Drawing for the job (mm, zero at the part's lowest x, y, z). A direction names the side the tool comes from. Round coordinates to 2 decimals unless told otherwise and drop trailing zeros. Write each loop counter-clockwise with the first axis right and the second up, starting at its lowest first coordinate (ties: lowest second). Pieces come first, ordered by that corner, then holes. Notation, with made-up numbers: M 18.25,72.25 L 48.25,72.25 A9 cw 48.25,87.25 Z; hole C 56,56.5 d5. An arc over 180 degrees is marked long. Use a Markdown table: item, result.
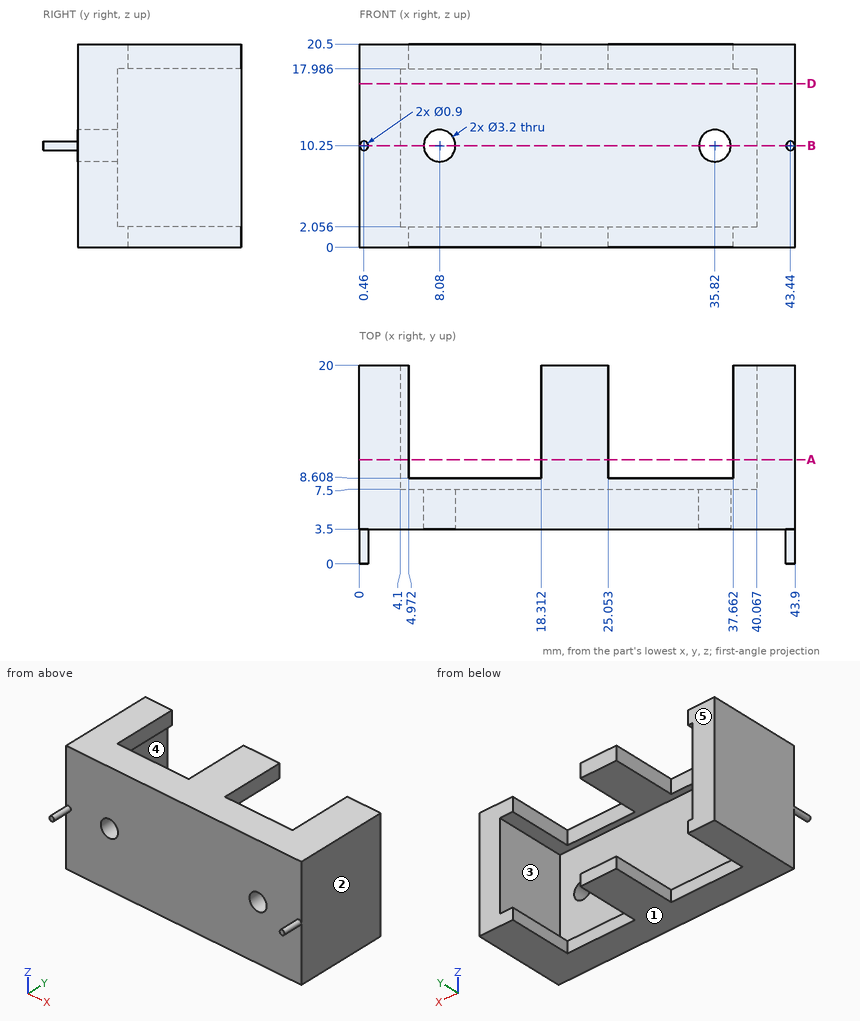
Q1. Cut at A-A on y = 10.5. Give the cut face in (x, z) (1 decimal).
Response values:
| item | result |
|---|---|
| outline | M 0,0 L 5,0 L 5,2.1 L 4.1,2.1 L 4.1,18 L 5,18 L 5,20.5 L 0,20.5 Z; M 18.3,0 L 25.1,0 L 25.1,2.1 L 18.3,2.1 Z; M 18.3,18 L 25.1,18 L 25.1,20.5 L 18.3,20.5 Z; M 37.7,0 L 43.9,0 L 43.9,20.5 L 37.7,20.5 L 37.7,18 L 40.1,18 L 40.1,2.1 L 37.7,2.1 Z |
Q2. Cut at B-B on z = 10.25. Count the separate pieces of the cut face and the enclosed holes in it.
Response values:
| item | result |
|---|---|
| separate pieces | 3 |
| enclosed holes | 0 |
Q3. Cut at D-D on z = 16.5. Give the cut face in (x, y).
Response values:
| item | result |
|---|---|
| outline | M 0,3.5 L 43.9,3.5 L 43.9,20 L 40.07,20 L 40.07,7.5 L 4.1,7.5 L 4.1,20 L 0,20 Z |
Q4. Two-plate mould, pull along Z, no slides. Class the marked faces 1, 2 and 3: +Z half, -Z half, draft (parallel to the pull), parting line (faces both ways), or undercut.
Response values:
| item | result |
|---|---|
| face 1 | -Z half |
| face 2 | draft |
| face 3 | undercut |
Q5. Drill centre lines: L1, parallel to X at y = 6.1, z = 10.25; L2, parallel to X at y = 12, z = 15.25; L3, parallel to Z at x = 39.5, y = 18.75 (1 decimal). Where is each one in solid material? Low to high.
Response values:
| item | result |
|---|---|
| L1 | x = 0 to 6.48, 9.68 to 34.22, 37.42 to 43.9 |
| L2 | x = 0 to 4.1, 40.07 to 43.9 |
| L3 | z = 0 to 2.1, 18 to 20.5 |
Q6. Drop flat-ended pins along their axis: P1, Ø12, axis at x = 24.5, z = 7.5, coming from the -Y side; P2, Ø1.9, axis at x = 8.08, z = 10.25, coming from the -Y side; P3, Ø0.6, axis at x = 9.5, z = 1, coming from the +Y side; P4, Ø5, axis at x = 23.5, z = 13.5, coming from the +Y side. Give the stop position or say it passes through.
Response values:
| item | result |
|---|---|
| P1 | stops at y = 3.5 |
| P2 | passes through |
| P3 | stops at y = 8.61 |
| P4 | stops at y = 7.5 |
Q7. Which spindle directions (+Z, -Z, +X, -X, +Y, -Y) get a long thin tool onto all of the face, cutting with end or side? Do the marked faces 4 and 5. Say none if no direction does.
Response values:
| item | result |
|---|---|
| face 4 | +Y |
| face 5 | +Z, -Z, +X, -X, +Y |
